```python
from build123d import *

# Parameters (mm, degrees)
F0_W            = 8
F0_H            = 17.5
F3_D            = 6
F4_T            = -2
F6_D            = 8
F6_COPIES_COUNT = 5
F7_SIZE         = 1


# Not quite as in the source:
# - a pattern or mirror of a feature is missing from the dataset's text; its kind, count and spacing are read off the source's solid


with BuildPart() as f1:
    # F0 (on Front) → F1 (revolve)
    with BuildSketch(Plane.XZ):
        with Locations((4, 8.75)):
            Rectangle(F0_W, F0_H)
    revolve(axis=Axis((4, 0, 0), (1, 0, 0)))

    # F3 (through all)
    with Locations(Plane(origin=(0, 0, 0), x_dir=(0, 1, 0), z_dir=(-1, 0, 0))):
        with Locations((0, 0)):
            Hole(F3_D / 2)

    # F4
    f4_openings = [f1.faces().sort_by_distance(p)[0] for p in [
        (8, 0, -17.005025),
    ]]
    offset(amount=F4_T, openings=f4_openings)

    # F6 (through all)
    with Locations(Plane(origin=(0, 0, 0), x_dir=(0, 1, 0), z_dir=(-1, 0, 0))):
        with Locations((0, -10)):
            f6 = Hole(F6_D / 2)

    # F6_copies: F6 ×5 about axis
    f6_copies_axis = Axis((0, 0, 0), (1, 0, 0))
    for i in range(1, F6_COPIES_COUNT):
        add(f6.rotate(f6_copies_axis, i * 360 / F6_COPIES_COUNT), mode=Mode.SUBTRACT)

    # F7
    f7_edges = [f1.edges().sort_by_distance(p)[0] for p in [
        (8, 0, -17.5),
    ]]
    chamfer(f7_edges, length=F7_SIZE)


solid = f1.part
```
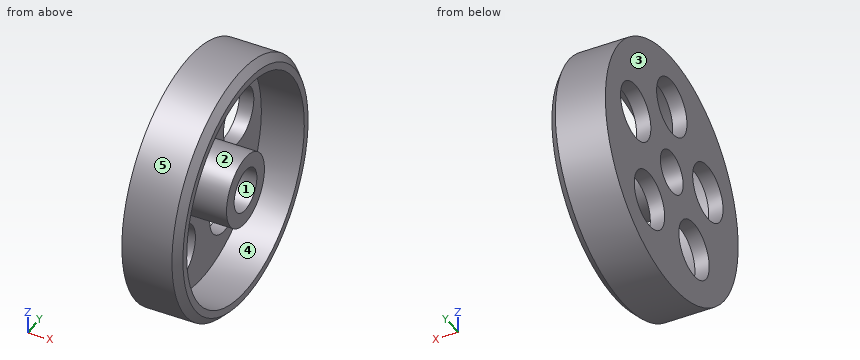
Source: CAD feature listing. Evaluate the final solid. Frame: model axes, mm. Face numbers are marked on the shaded views. A direction names the side the tool comes from. Coordinates: 2 decimals unless noted, no trailing zeros. Loops run counter-clockwise (first coordinate to the right, second up) from the corner with the lowest first, then second, coordinate; pieces in that order, holes last. Notation, with made-up numbers: M 42.5,10 L 97.5,10 A20 cw 97.5,36 Z; hole C 49.5,-12 d8. An arc over 180 degrees is marked long. Use a Markdown table: item, result. Add a question column.
Q1. Section query C-C, the plane z = 0. Return loops of the section in (x, y).
Q2. First-contact query: pin 1 (2 mm diameter, centred on y = 11, z = 4.5, fed in from +X); pin 2 (4 mm diameter, centred on x = 4, y = 4.5, fed in from +Z); pin 3 (3 mm diameter, centred on x = 4.5, z = -7, fed in from +Y); pin 4 (8 mm diameter, centred on y = 3, z = -11, fed in from +X). Flat tips, straight axial feed; report the tip coordinate or a pass-through.
Q3. Access query for the marked faces 1 and 2. Directions: +Z, -Z, +X, -X, +Y, -Y. A direction counts if a zero-diameter tool reaches every point of the face in a straight line with its end or side. Return the directions, or none.
Q4. Material intervals for L1, parallel to Z at x = 1.15, y = 0; L2, parallel to Z at x = 5.25, y = 0; L3, parallel to Y at x = 1.75, z = 5, sorted ascending.
Q5. Section query B-B, the plane x = 5.25. Return loops of the section in (y, z), and give its area (3 significant figures).
Q6. Draft query along Z for the marked faces 3, 4 and 5. Return one class per face: pulls with the +Z half, pulls with the -Z half, needs draft (parallel to the pull), parting line crosses it, or undercut.
Q7. Section query A-A, the plane y = 0. Return loops of the section in (x, z), and give its area (3 significant figures).
Q8. Section query D-D, the plane z = -11. State how many separate pieces and enclosed holes the cut face has, and give its area (3 significant figures).
Result:
| question | item | result |
|---|---|---|
| 1 | outline | M 0,-17.5 L 7,-17.5 L 8,-16.5 L 8,-15.5 L 2,-15.5 L 2,-12.05 L 0,-12.05 Z; M 0,-6.97 L 2,-6.97 L 2,-5 L 8,-5 L 8,-3 L 0,-3 Z; M 0,3 L 8,3 L 8,5 L 2,5 L 2,6.97 L 0,6.97 Z; M 0,12.05 L 2,12.05 L 2,15.5 L 8,15.5 L 8,16.5 L 7,17.5 L 0,17.5 Z |
| 2 | pin 1 | passes through |
| 2 | pin 2 | stops at z = 17.32 |
| 2 | pin 3 | stops at y = 16.61 |
| 2 | pin 4 | stops at x = 2 |
| 3 | face 1 | +X, -X |
| 3 | face 2 | +X |
| 4 | L1 | z = -17.5 to -3, 3 to 6, 14 to 17.5 |
| 4 | L2 | z = -17.5 to -15.5, -5 to -3, 3 to 5, 15.5 to 17.5 |
| 4 | L3 | y = -16.77 to -13.03, -6 to 6, 13.03 to 16.77 |
| 5 | outline | C 0,0 d35; C 0,0 d10; hole C 0,0 d31; hole C 0,0 d6 |
| 5 | area | 258 mm2 |
| 6 | face 3 | needs draft |
| 6 | face 4 | undercut |
| 6 | face 5 | parting line crosses it |
| 7 | outline | M 0,-17.5 L 7,-17.5 L 8,-16.5 L 8,-15.5 L 2,-15.5 L 2,-5 L 8,-5 L 8,-3 L 0,-3 Z; M 0,3 L 8,3 L 8,5 L 2,5 L 2,6 L 0,6 Z; M 0,14 L 2,14 L 2,15.5 L 8,15.5 L 8,16.5 L 7,17.5 L 0,17.5 Z |
| 7 | area | 89.0 mm2 |
| 8 | separate pieces | 3 |
| 8 | enclosed holes | 0 |
| 8 | area | 63.5 mm2 |
